from build123d import *

# Parameters (mm, degrees)
SKETCH1_R             = 130
BOSS_EXTRUDE1_DEPTH   = 190
FILLET1_R             = 25
SKETCH2_R             = 36.5
BOSS_EXTRUDE2_DEPTH   = 20
M8_TAPPED_HOLE2_D     = 6.8
M8_TAPPED_HOLE2_DEPTH = 17.707073895
M8_TAPPED_HOLE2_TIP   = 2.042926105
SKETCH8_R             = 36.5
BOSS_EXTRUDE3_DEPTH   = 100
CHAMFER1_SIZE         = 10


with BuildPart() as part:
    # Sketch1 → Boss-Extrude1 (new body)
    with BuildSketch(Plane(origin=(0, 0, 0), x_dir=(1, 0, 0), z_dir=(0, 1, 0))):
        Circle(SKETCH1_R)
    extrude(amount=BOSS_EXTRUDE1_DEPTH)

    # Fillet1
    fillet1_edges = [part.edges().sort_by_distance(p)[0] for p in [
        (-130, 0, 0),
        (-130, 190, 0),
    ]]
    fillet(fillet1_edges, radius=FILLET1_R)

    # Sketch2 → Boss-Extrude2 (add)
    with BuildSketch(Plane.XZ):
        Circle(SKETCH2_R)
    extrude(amount=BOSS_EXTRUDE2_DEPTH)

    # M8 Tapped Hole2
    with Locations(Plane(origin=(0, 0, 0), x_dir=(-1, 0, 0), z_dir=(0, -1, 0))):
        with Locations((0, -95), (-95, 0), (0, 95), (95, 0)):
            Hole(M8_TAPPED_HOLE2_D / 2, depth=M8_TAPPED_HOLE2_DEPTH)
            with Locations((0, 0, -(M8_TAPPED_HOLE2_DEPTH + M8_TAPPED_HOLE2_TIP / 2))):  # 118° drill point
                Cone(0, M8_TAPPED_HOLE2_D / 2, M8_TAPPED_HOLE2_TIP, mode=Mode.SUBTRACT)

    # Sketch8 → Boss-Extrude3 (add)
    with BuildSketch(Plane(origin=(0, 190, 0), x_dir=(1, 0, 0), z_dir=(0, 1, 0))):
        Circle(SKETCH8_R)
    extrude(amount=BOSS_EXTRUDE3_DEPTH)

    # Chamfer1
    chamfer1_edges = [part.edges().sort_by_distance(p)[0] for p in [
        (-36.5, 290, 0),
    ]]
    chamfer(chamfer1_edges, length=CHAMFER1_SIZE)


solid = part.part
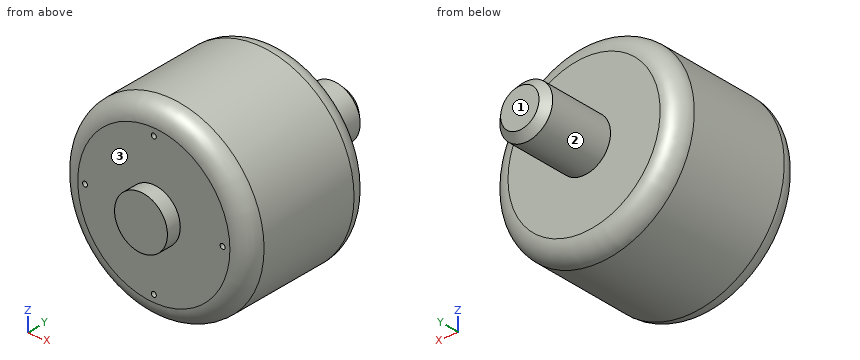
CAD build for the part. Positions are in the model's coordinates, mm. Face numbers are marked on the shaded views. A direction names the side the tool comes from. Coordinates: 2 decimals unless noted, no trailing zeros. Loops run counter-clockwise (first coordinate to the right, second up) from the corner with the lowest first, then second, coordinate; pieces in that order, holes last. Notation, with made-up numbers: (72.5, 28) - (90.5, 28) arc R28 cw to (90.5, 47) - close; hole circle Ø11 at (36, 31.5). An arc over 180 degrees is marked (long way). Use one line per item in the form item = value. Start each with the question number.
1) Drill centre lines: L1, parallel to Z at x = 0, y = 10.75; L2, parallel to Y at x = 31, z = -20; L3, parallel to Z at x = 0, y = 4. Where is each one in solid material? Low to high. Write a range as from..to.
2) Band-saw the part on B-B (y = 104). Give the cut face in (x, z), and give its area (3 significant figures).
3) Tool access for the marked faces 1, 2 and 3: list every direction of +Z, -Z, +X, -X, +Y, -Y with a clear straight run to the whole face (end or side of a thin tool).
4) Band-saw the part on A-A (y = 243). Give the cut face in (x, z).
5) Flat gauge pins, fed straight in: pin 1 (10 mm diameter, centred on y = 137.5, z = 73.5, fed in from -X); pin 2 (3 mm diameter, centred on x = 44, y = 143, fed in from -Z); pin 3 (4 mm diameter, centred on x = 95, z = 0, fed in from +Y). Where does each tip first touch, or does it go through?
Check values:
q1.L1 = -125.54..-98.4, -91.6..91.6, 98.4..125.54
q1.L2 = 0..190
q1.L3 = -118.56..-98.4, -91.6..91.6, 98.4..118.56
q2.outline = circle Ø260 at (0, 0)
q2.area = 53,100 mm2
q3.face_1 = +Z, -Z, +X, -X, +Y
q3.face_2 = +Y
q3.face_3 = -Y
q4.outline = circle Ø73 at (0, 0)
q5.pin_1 = -110.49
q5.pin_2 = -122.86
q5.pin_3 = 190
